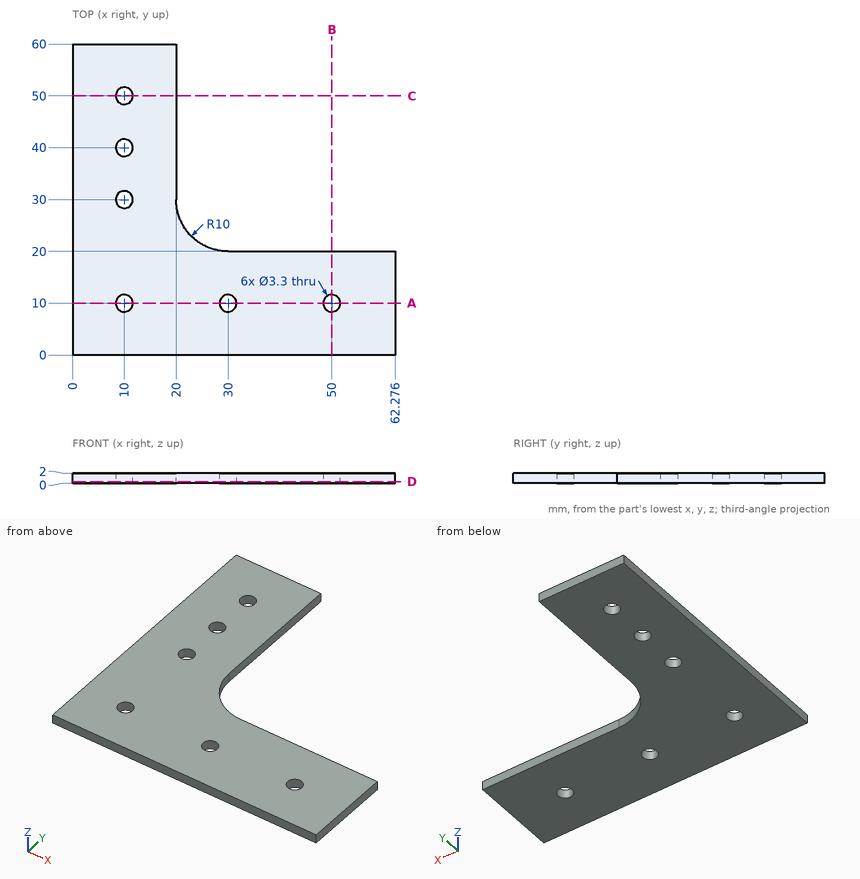
For this review, use the dimensioned drawing (mm, ordinates from the lowest corner) and the shaded views. Round coordinates to 2 decimals unless told otherwise and drop trailing zeros. Loops run counter-clockwise (first coordinate to the right, second up) from the corner with the lowest first, then second, coordinate; pieces in that order, holes last. Notation, with made-up numbers: (41.25, -1.75) -> (92.25, -1.75) arc R9 ccw to (92.25, 10.25) -> close; hole circle Ø1 at (7.25, -13.75). An arc over 180 degrees is marked (long way). Write item = value, one per line. Start each with the question number.
Item 1: Take a section at D-D on z = 0.35. Give the boundary of the cut face in (x, y).
Item 2: Take a section at A-A on y = 10. Give the boundary of the cut face in (x, z), plus the area to 3 significant figures.
Item 3: Take a section at B-B on x = 50. Give the boundary of the cut face in (y, z), plus the area to 3 significant figures.
Item 4: To check wall thickness, follow L1, parallel to Y at x = 10, z = 1.6; L2, parallel to Y at x = 50, z = 1.3; L3, parallel to X at y = 52, z = 1.65. State the ranges of each line that lie inside material, in increasing order.
Result:
q1.outline = (0, 0) -> (62.28, 0) -> (62.28, 20) -> (30, 20) arc R10 cw to (20, 30) -> (20, 60) -> (0, 60) -> close; hole circle Ø3.3 at (10, 10); hole circle Ø3.3 at (10, 30); hole circle Ø3.3 at (10, 40); hole circle Ø3.3 at (10, 50); hole circle Ø3.3 at (30, 10); hole circle Ø3.3 at (50, 10)
q2.outline = (0, 0) -> (8.35, 0) -> (8.35, 2) -> (0, 2) -> close; (11.65, 0) -> (28.35, 0) -> (28.35, 2) -> (11.65, 2) -> close; (31.65, 0) -> (48.35, 0) -> (48.35, 2) -> (31.65, 2) -> close; (51.65, 0) -> (62.28, 0) -> (62.28, 2) -> (51.65, 2) -> close
q2.area = 105 mm²
q3.outline = (0, 0) -> (8.35, 0) -> (8.35, 2) -> (0, 2) -> close; (11.65, 0) -> (20, 0) -> (20, 2) -> (11.65, 2) -> close
q3.area = 33.4 mm²
q4.L1 = 0 to 8.35, 11.65 to 28.35, 31.65 to 38.35, 41.65 to 48.35, 51.65 to 60
q4.L2 = 0 to 8.35, 11.65 to 20
q4.L3 = 0 to 20
